```python
from build123d import *

# Parameters (mm, degrees)
SKETCH_W     = 62.5
SKETCH_H     = 95
PAD_DEPTH    = 10
PAD001_DEPTH = 7
POCKET_DEPTH = 3
SKETCH003_W  = 2
SKETCH003_H  = 21
PAD002_DEPTH = 4.8
FILLET_R     = 5


with BuildPart() as part:
    # Sketch → Pad (new body)
    with BuildSketch(Plane.XY):
        with Locations((31.25, -47.5)):
            Rectangle(SKETCH_W, SKETCH_H)
    extrude(amount=PAD_DEPTH)

    # Sketch001 (on Face6 of Pad) → Pad001 (join)
    with BuildSketch(Plane.XY.offset(10)):
        with BuildLine():
            ThreePointArc((66.035523, -3.535545), (66.035539, 3.535528), (58.964466, 3.535534))
            ThreePointArc((54.5, 0), (57.061192, 1.352376), (58.964466, 3.535534))
            Line((54.5, 0), (62.5, -8))
            ThreePointArc((66.035523, -3.535545), (63.868245, -5.451384), (62.5, -8))
        make_face()
    extrude(amount=-PAD001_DEPTH)

    # Sketch002 (on Face2 of Pad001) → Pocket (cut)
    with BuildSketch(Plane(origin=(0, 0, 0), x_dir=(1, 0, 0), z_dir=(0, 0, -1))):
        with BuildLine():
            Line((54.5, 0), (62.5, 0))
            Line((62.5, 0), (62.5, 8))
            ThreePointArc((62.5, 8), (63.868245, 5.451384), (66.035523, 3.535545))
            ThreePointArc((58.964466, -3.535534), (66.035539, -3.535528), (66.035523, 3.535545))
            ThreePointArc((58.964466, -3.535534), (57.061192, -1.352376), (54.5, 0))
        make_face()
    extrude(amount=-POCKET_DEPTH, mode=Mode.SUBTRACT)

    # Sketch003 (on Face3 of Pocket) → Pad002 (join)
    with BuildSketch(Plane(origin=(0, 0, 0), x_dir=(1, 0, 0), z_dir=(0, 0, -1))):
        with Locations((10, 56)):
            Rectangle(SKETCH003_W, SKETCH003_H)
    extrude(amount=PAD002_DEPTH)

    # Fillet
    fillet_edges = [part.edges().sort_by_distance(p)[0] for p in [
        (0, 0, 5),
        (0, -95, 5),
        (62.5, -95, 5),
    ]]
    fillet(fillet_edges, radius=FILLET_R)


solid = part.part
```
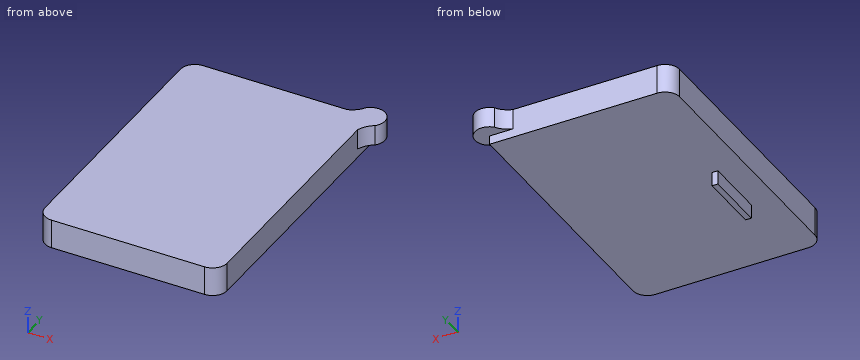
Input: part model. Units: mm. Frame: model coordinates. Give positions to 0.01 mm unless a question says otherwise; leave off trailing zeros. Loops run counter-clockwise (first coordinate to the right, second up) from the corner with the lowest first, then second, coordinate; pieces in that order, holes last.
1) Section query A-A on y = -56.5. Return the cut outline in (x, z), and give its area (3 significant figures).
A:
outline: (0, 0) - (9, 0) - (9, -4.8) - (11, -4.8) - (11, 0) - (62.5, 0) - (62.5, 10) - (0, 10) - close
area: 635 mm2
2) Line query: L1, parallel to X at y = -51, z = 3; L2, parallel to Z at x = 4, y = -16.5; L3, parallel to X at y = -65, z = -0.25. Output: solid intervals per line, ascending.
A:
L1: x = 0 to 62.5
L2: z = 0 to 10
L3: x = 9 to 11
3) Contact query for flat-ended pins moving along their axis: pin 1 (2 mm diameter, centred on x = 39, y = -7.5, fed in from -Z); pin 2 (8 mm diameter, centred on y = -61.5, z = -1, fed in from +X); pin 3 (4 mm diameter, centred on y = -52, z = -2.5, fed in from +X). Output: stop coordinate, or through.
A:
pin 1: stops at z = 0
pin 2: stops at x = 62.5
pin 3: stops at x = 11
4) Section query B-B on z = 6.25. Return the cut outline in (x, y), and give its area (4 significant figures).
A:
outline: (0, -90) arc R5 ccw to (5, -95) - (57.5, -95) arc R5 ccw to (62.5, -90) - (62.5, -8) arc R8.21 cw to (66.04, -3.54) arc R5 ccw to (58.96, 3.54) arc R7.92 cw to (54.5, 0) - (5, 0) arc R5 ccw to (0, -5) - close
area: 5,985 mm2
5) Section query D-D on y = -11.5. Return the cut outline in (x, z).
A:
outline: (0, 0) - (62.5, 0) - (62.5, 10) - (0, 10) - close
6) Section query C-C on x = 6. Return the cut outline in (y, z), and give its area (3 significant figures).
A:
outline: (-95, 0) - (0, 0) - (0, 10) - (-95, 10) - close
area: 950 mm2
